Part model, mm, in its own coordinate system. A direction names the side the tool comes from. Round coordinates to 2 decimals unless told otherwise and drop trailing zeros. Loops run counter-clockwise (first coordinate to the right, second up) from the corner with the lowest first, then second, coordinate; pieces in that order, holes last. Notation, with made-up numbers: (-6.5, 45) -> (37.5, 45) arc R33 ccw to (37.5, 73) -> close; hole circle Ø6 at (20, -13). An arc over 180 degrees is marked (long way). Answer as a JSON object with one key per item and string values. Group by question number.
from build123d import *

# Parameters (mm, degrees)
BOSS_EXTRUDE4_DEPTH                      = 25.4
SKETCH5_R                                = 1.4224
CAGE_MOUNTING_HOLE_4_40_TAPPED_DEPTH     = 3.81
BOSS_EXTRUDE5_DEPTH                      = 3.81
SKETCH7_R                                = 1.4224
BASE_MOUNTING_HOLES_4_40_CLEARANCE_DEPTH = 3.81


with BuildPart() as part:
    # Sketch4 → Boss-Extrude4 (new body)
    with BuildSketch(Plane(origin=(0, 0, 0), x_dir=(1, 0, 0), z_dir=(0, 1, 0))):
        Polygon((-2.732505263, 2.4892), (-2.732505263, 10.1092), (-0.192505263, 10.1092), (-0.192505263, 2.4892), (2.347494737, 2.4892), (2.347494737, -0.0508), (9.967494737, -0.0508), (9.967494737, -2.5908), (2.347494737, -2.5908), (-2.732505263, -2.5908), align=None)
    extrude(amount=BOSS_EXTRUDE4_DEPTH)

    # Sketch5 → Cage Mounting Hole (4-40 Tapped) (cut)
    with BuildSketch(Plane(origin=(0, 25.4, 0), x_dir=(1, 0, 0), z_dir=(0, 1, 0))):
        with Locations((-0.192505263, -0.0508)):
            Circle(SKETCH5_R)
    extrude(amount=-CAGE_MOUNTING_HOLE_4_40_TAPPED_DEPTH, mode=Mode.SUBTRACT)

    # Sketch6 → Boss-Extrude5 (add)
    with BuildSketch(Plane.XZ):
        Polygon((9.967494737, 2.5908), (9.967494737, 10.2108), (-10.352505263, 10.2108), (-10.352505263, -10.1092), (-2.732505263, -10.1092), (-2.732505263, 2.5908), align=None)
    extrude(amount=-BOSS_EXTRUDE5_DEPTH)

    # Sketch7 → Base Mounting Holes (4-40 Clearance) (cut)
    with BuildSketch(Plane(origin=(0, 3.81, 0), x_dir=(1, 0, 0), z_dir=(0, 1, 0))):
        with Locations((-6.542505263, 3.7592)):
            Circle(SKETCH7_R)
        with Locations((3.617494737, -6.4008)):
            Circle(SKETCH7_R)
    extrude(amount=-BASE_MOUNTING_HOLES_4_40_CLEARANCE_DEPTH, mode=Mode.SUBTRACT)


solid = part.part
Item 1: Drill centre lines: line 1 (Y direction, x = 6.25, z = 8); line 2 (X direction, y = 1.5, z = -6); line 3 (X direction, y = 19.25, z = -6.75). Where is each one in solid material? Low to high.
Item 2: Drop flat-ended pins along their axis: pin 1 Ø5 at (y, z) = (11.5, -5) entering from -X; pin 2 Ø1.3 at (y, z) = (16.5, -1) entering from +X; pin 3 Ø8.5 at (x, y) = (5, 18.5) entering from -Z. Give the stop position or say it passes through.
Item 3: Band-saw the part on C-C, the plane y = 22. List the corners of the cut face in (x, z).
Item 4: Band-saw the part on D-D, the plane z = -6. List the corners of the cut face in (x, y).
Item 5: Two-plate mould, pull along X, no slides. Class faces 1 (the face through (2, 25.4, -2)), 2 (the face through (2.347, 13, -1)), 3 (the face through (0.57, 23.52, -1.15)): pulls with the +X half, pulls with the -X half, needs draft (parallel to the pull), parting line crosses it, or undercut.
Item 6: Band-saw the part on A-A, the plane z = 6. List the corners of the cut face in (x, y), plus the area to 3 significant figures.
Item 7: Band-saw the part on B-B, the plane x = 3.5. List the corners of the cut face in (y, z).
Item 8: Which spindle directions (+Z, -Z, +X, -X, +Y, -Y) get a long thin tool onto all of the face, cutting with end or side? Do faces 4 (the face through (6, 13, 0.051)), 5 (the face through (-2.733, 14, -4)), 6 (the face through (0, 21.59, 0)). Say none if no direction does.
Entries:
{
 "1": {"line 1": "0 to 3.81", "line 2": "-10.35 to -0.19", "line 3": "-2.73 to -0.19"},
 "2": {"pin 1": "x = -2.73", "pin 2": "x = 2.35", "pin 3": "z = -2.49"},
 "3": {"outline": "(-2.73, -10.11) -> (-0.19, -10.11) -> (-0.19, -2.49) -> (2.35, -2.49) -> (2.35, 0.05) -> (9.97, 0.05) -> (9.97, 2.59) -> (-2.73, 2.59) -> close; hole circle Ø2.84 at (-0.19, 0.05)"},
 "4": {"outline": "(-10.35, 0) -> (-0.19, 0) -> (-0.19, 25.4) -> (-2.73, 25.4) -> (-2.73, 3.81) -> (-10.35, 3.81) -> close"},
 "5": {"face 1": "needs draft", "face 2": "pulls with the +X half", "face 3": "undercut"},
 "6": {"outline": "(-10.35, 0) -> (2.25, 0) -> (2.25, 3.81) -> (-10.35, 3.81) -> close; (4.98, 0) -> (9.97, 0) -> (9.97, 3.81) -> (4.98, 3.81) -> close", "area": "67.0 mm²"},
 "7": {"outline": "(0, 0.05) -> (25.4, 0.05) -> (25.4, 2.59) -> (3.81, 2.59) -> (3.81, 4.98) -> (0, 4.98) -> close; (0, 7.82) -> (3.81, 7.82) -> (3.81, 10.21) -> (0, 10.21) -> close"},
 "8": {"face 4": "-Z, +X, +Y, -Y", "face 5": "+Z, -Z, -X, +Y", "face 6": "+Y"}
}
